Design review of the part built by this model. Coordinates are the model's own, in mm. Face numbers are marked on the shaded views. A direction names the side the tool comes from. Round coordinates to 2 decimals unless told otherwise and drop trailing zeros. Order: outer loops, then holes, each group sorted by start corner. A loop starts at its lowest first (then second) coordinate and runs counter-clockwise, first axis right, second up.
from build123d import *

# Parameters (mm, degrees)
SKETCH1_W           = 18
SKETCH1_H           = 18
BOSS_EXTRUDE1_DEPTH = 20
SKETCH2_R           = 4.15
CUT_EXTRUDE1_DEPTH  = 21
SKETCH3_R           = 1.5
CUT_EXTRUDE2_DEPTH  = 19
SKETCH4_W           = 18
SKETCH4_H           = 45
BOSS_EXTRUDE2_DEPTH = 2
SKETCH5_R           = 1.5
CUT_EXTRUDE3_DEPTH  = 21
FILLET1_R           = 7
CUT_EXTRUDE4_DEPTH  = 33.5


with BuildPart() as part:
    # Sketch1 → Boss-Extrude1 (new body)
    with BuildSketch(Plane(origin=(0, 0, 0), x_dir=(1, 0, 0), z_dir=(0, 1, 0))):
        with Locations((0, 9)):
            Rectangle(SKETCH1_W, SKETCH1_H)
    extrude(amount=BOSS_EXTRUDE1_DEPTH)

    # Sketch2 → Cut-Extrude1 (cut, through all)
    with BuildSketch(Plane(origin=(0, 20, 0), x_dir=(1, 0, 0), z_dir=(0, 1, 0))):
        with Locations((0, 6.5)):
            Circle(SKETCH2_R)
        with BuildLine():
            Line((1, 10.527716475), (1, 18))
            Line((1, 18), (0, 18))
            Line((0, 18), (-1, 18))
            Line((-1, 18), (-1, 10.527716475))
            ThreePointArc((-1, 10.527716475), (0, 2.35), (1, 10.527716475))
        make_face()
    extrude(amount=-CUT_EXTRUDE1_DEPTH, mode=Mode.SUBTRACT)

    # Sketch3 → Cut-Extrude2 (cut, through all)
    with BuildSketch(Plane(origin=(9, 0, 0), x_dir=(0, 0, -1), z_dir=(1, 0, 0))):
        with Locations((15.5, 16)):
            Circle(SKETCH3_R)
        with Locations((15.5, 4)):
            Circle(SKETCH3_R)
    extrude(amount=-CUT_EXTRUDE2_DEPTH, mode=Mode.SUBTRACT)

    # Sketch4 → Boss-Extrude2 (add)
    with BuildSketch(Plane.XY):
        with Locations((0, 10)):
            Rectangle(SKETCH4_W, SKETCH4_H)
    extrude(amount=BOSS_EXTRUDE2_DEPTH)

    # Sketch5 → Cut-Extrude3 (cut, through all)
    with BuildSketch(Plane.XY.offset(2)):
        with Locations((0, 28)):
            Circle(SKETCH5_R)
        with Locations((0, -8)):
            Circle(SKETCH5_R)
    extrude(amount=-CUT_EXTRUDE3_DEPTH, mode=Mode.SUBTRACT)

    # Fillet1
    fillet1_edges = [part.edges().sort_by_distance(p)[0] for p in [
        (9, -12.5, 1),
        (9, 32.5, 1),
        (-9, 32.5, 1),
        (-9, -12.5, 1),
    ]]
    fillet(fillet1_edges, radius=FILLET1_R)

    # Sketch6 → Cut-Extrude4 (cut, through all)
    with BuildSketch(Plane.XZ):
        with BuildLine():
            Line((-3.5, -13.693747285), (-3.5, -18))
            Line((-3.5, -18), (-9, -18))
            Line((-9, -18), (-9, 0))
            Line((-9, 0), (-8, 0))
            Line((-8, 0), (-8, -6.5))
            ThreePointArc((-8, -6.5), (-6.782329983, -10.742640687), (-3.5, -13.693747285))
        make_face()
        with BuildLine():
            Line((8, 0), (8, -6.5))
            ThreePointArc((8, -6.5), (6.782329983, -10.742640687), (3.5, -13.693747285))
            Line((3.5, -13.693747285), (3.5, -18))
            Line((3.5, -18), (9, -18))
            Line((9, -18), (9, 0))
            Line((9, 0), (8, 0))
        make_face()
    extrude(amount=-CUT_EXTRUDE4_DEPTH, mode=Mode.SUBTRACT)


solid = part.part
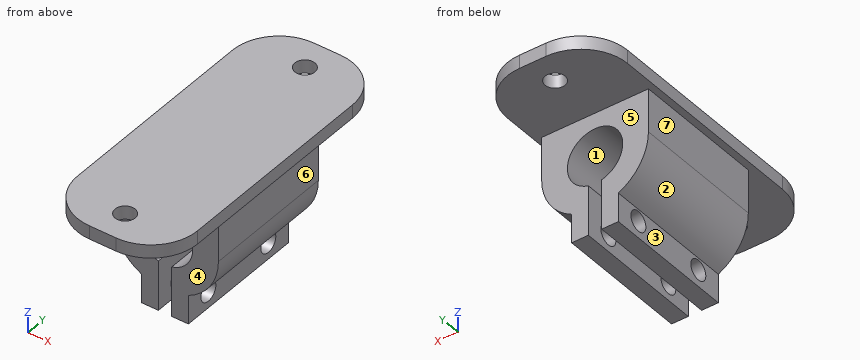
1) The part is to be moulded in two halves that separate along Z. For the marked faces 1, 2 and 3, say which applies: released by +Z, released by -Z, zero draft, split by the parting line, or undercut.
Results:
face 1: undercut
face 2: released by -Z
face 3: zero draft
2) For the marked faces 4, 5, 6 and 7, list the 3-axis set-ups (+Z, -Z, +X, -X, +Y, -Y) from which the entire face can be reached by the end or side of a thin tool; tool diameter is ignored.
Results:
face 4: -Z, +X, -X, -Y
face 5: -Z, +X, -X, +Y
face 6: -Z, +X, +Y, -Y
face 7: -Z, -X, +Y, -Y
3) Take a section at C-C on x = 2.75. Give the boundary of the cut face in (y, z), plus the area to 3 significant figures.
Results:
outline: (-12.46, 0) - (0, 0) - (0, -3.39) - (20, -3.39) - (20, 0) - (32.46, 0) - (32.46, 2) - (-12.46, 2) - close; (0, -18) - (20, -18) - (20, -9.61) - (0, -9.61) - close; hole circle Ø3 at (4, -15.5); hole circle Ø3 at (16, -15.5)
area: 311 mm2
4) To check wall thickness, follow line 1 along Y through (x, z) = (0, 0.6); line 2 along Y through (x, z) = (-2.9, -15.5); line 3 along X through (y, z) = (11.75, -6.5). State the ranges of each line that lie inside material, in increasing order.
Results:
line 1: y = -12.5 to -9.5, -6.5 to 26.5, 29.5 to 32.5
line 2: y = 0 to 2.5, 5.5 to 14.5, 17.5 to 20
line 3: x = -8 to -4.15, 4.15 to 8
5) Take a section at B-B on z = -15.5. Give the boundary of the cut face in (x, y).
Results:
outline: (-3.5, 0) - (-1, 0) - (-1, 2.5) - (-3.5, 2.5) - close; (-3.5, 5.5) - (-1, 5.5) - (-1, 14.5) - (-3.5, 14.5) - close; (-3.5, 17.5) - (-1, 17.5) - (-1, 20) - (-3.5, 20) - close; (1, 0) - (3.5, 0) - (3.5, 2.5) - (1, 2.5) - close; (1, 5.5) - (3.5, 5.5) - (3.5, 14.5) - (1, 14.5) - close; (1, 17.5) - (3.5, 17.5) - (3.5, 20) - (1, 20) - close
6) Take a section at D-D on z = -11.25. Give the boundary of the cut face in (x, y), plus the area to 3 significant figures.
Results:
outline: (-6.44, 0) - (-1, 0) - (-1, 20) - (-6.44, 20) - close; (1, 0) - (6.44, 0) - (6.44, 20) - (1, 20) - close
area: 217 mm2
7) Take a section at A-A on x = 0. Give the boundary of the cut face in (y, z), plus the area to 3 significant figures.
Results:
outline: (-12.5, 0) - (-9.5, 0) - (-9.5, 2) - (-12.5, 2) - close; (-6.5, 0) - (0, 0) - (0, -2.35) - (20, -2.35) - (20, 0) - (26.5, 0) - (26.5, 2) - (-6.5, 2) - close; (29.5, 0) - (32.5, 0) - (32.5, 2) - (29.5, 2) - close
area: 125 mm2
8) Clearance check with flat-ended pins moving along their axes: P1, Ø6, axis at y = 11, z = -14.5, coming from the -X side (3 decimals); P2, Ø3.5, axis at y = 11, z = -15, coming from the -X side; P3, Ø2.5, axis at y = 16, z = -15.5, coming from the +X side; P4, Ø6, axis at x = -7, z = -9, coming from the -Y side. State where each tip first meets the part, or that it passes through.
Results:
P1: stops at x = -6.245
P2: stops at x = -4.29
P3: passes through
P4: stops at y = 0
